Here's the drawing with two shaded views (mm, measured from the low corner). I have some questions. A direction names the side the tool comes from. Give positions to 0.01 mm unless a question says otherwise; leave off trailing zeros. Write each loop counter-clockwise with the first axis right and the second up, starting at its lowest first coordinate (ties: lowest second). Pieces come first, ordered by that corner, then holes. Notation, with made-up numbers: (42.25, 74.5) - (89.25, 74.5) arc R28 ccw to (89.25, 112.5) - close; hole circle Ø8 at (27, -15). An arc over 180 degrees is marked (long way). Answer as a JSON object with one key per item and string values. Group by question number.
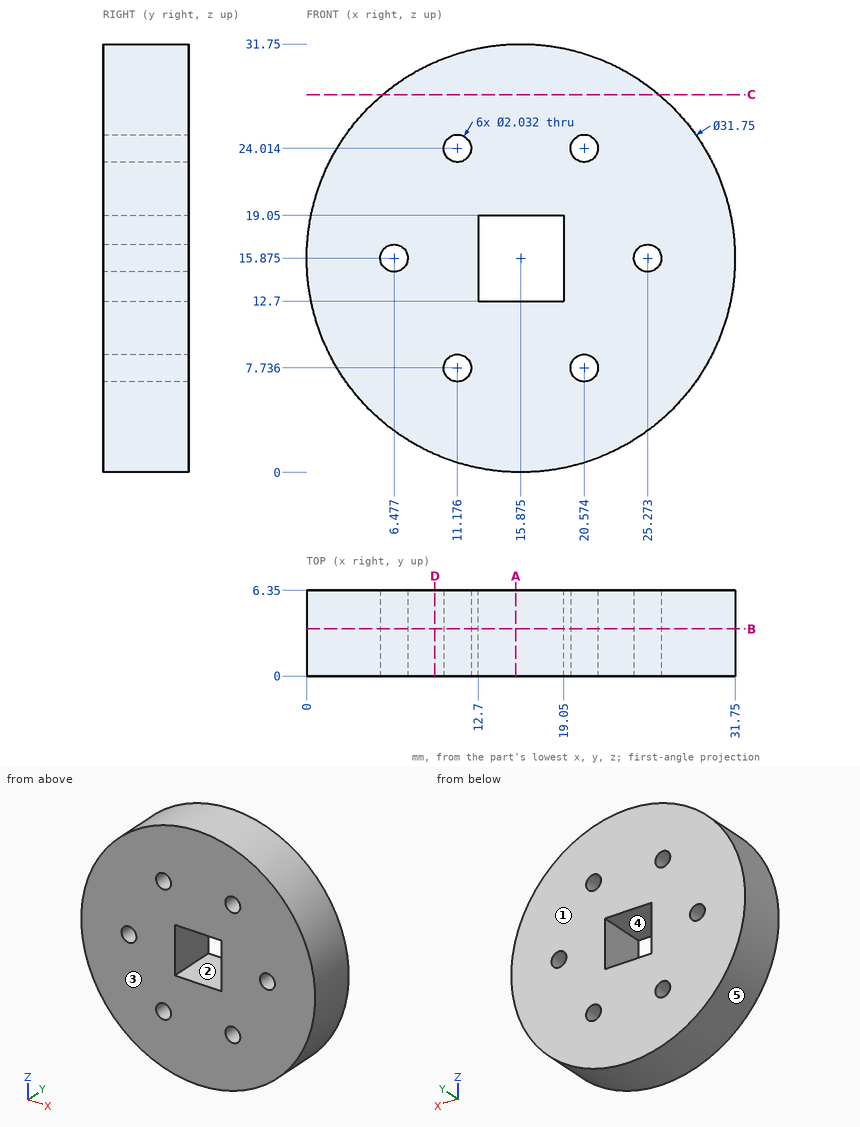
(1) I want a section at C-C, the plane z = 28. Please give me the cut outline in (x, y), and give its area (3 significant figures).
(2) For the marked faces 1 and 2, which set-ups out of +Z, -Z, +X, -X, +Y, -Y let a thin tool reach every point of the face, with its end or its side?
(3) I want a section at B-B, the plane y = 3.5. Please give me the cut outline in (x, z) (3 decimals), and give its area (3 significant figures).
(4) I want a section at A-A, the plane x = 15.5. Please give me the cut outline in (y, z).
(5) I need wall thicknesses on L1, parallel to X at y = 3.5, z = 16; L2, parallel to Z at x = 11, y = 5; L3, parallel to Z at x = 21, y = 2.75. Which ranges of each line are inside material? Lowest first, please.
(6) Will this pin go through, and if not, where does the flat tip stop? P1, Ø2, axis at x = 21.5, y = 3, coming from the +Z side.
(7) I want a section at D-D, the plane x = 9.5. Please give me the cut outline in (y, z), and give its area (3 significant figures).
(8) If we mould it in two halves opening along Z, with no side actions, what happens to the marked faces 3, 4 and 5? For each: +Z half, -Z half, draft (parallel to the pull), parting line (faces both ways), or undercut.
Entries:
{
 "1": {"outline": "(5.63, 0) - (26.12, 0) - (26.12, 6.35) - (5.63, 6.35) - close", "area": "130 mm^2"},
 "2": {"face 1": "+Z, -Z, +X, -X, +Y", "face 2": "+Y, -Y"},
 "3": {"outline": "circle Ø31.75 at (15.875, 15.875); hole circle Ø2.032 at (6.477, 15.875); hole circle Ø2.032 at (11.176, 7.736); hole circle Ø2.032 at (11.176, 24.014); hole (12.7, 12.7) - (19.05, 12.7) - (19.05, 19.05) - (12.7, 19.05) - close; hole circle Ø2.032 at (20.574, 7.736); hole circle Ø2.032 at (20.574, 24.014); hole circle Ø2.032 at (25.273, 15.875)", "area": "732 mm^2"},
 "4": {"outline": "(0, 0) - (6.35, 0) - (6.35, 12.7) - (0, 12.7) - close; (0, 19.05) - (6.35, 19.05) - (6.35, 31.75) - (0, 31.75) - close"},
 "5": {"L1": "0 to 5.47, 7.49 to 12.7, 19.05 to 24.26, 26.28 to 31.75", "L2": "0.77 to 6.74, 8.74 to 23.01, 25.01 to 30.98", "L3": "0.85 to 6.81, 8.66 to 23.09, 24.94 to 30.9"},
 "6": {"P1": "z = 31.06"},
 "7": {"outline": "(0, 1.34) - (6.35, 1.34) - (6.35, 30.41) - (0, 30.41) - close", "area": "185 mm^2"},
 "8": {"face 3": "draft", "face 4": "undercut", "face 5": "parting line"}
}
